from build123d import *

# Parameters (mm, degrees)
SKETCH2_R           = 5.9
BOSS_EXTRUDE1_DEPTH = 10
SKETCH3_R           = 2.075
CUT_EXTRUDE1_DEPTH  = 11
SKETCH4_W           = 11.8
SKETCH4_H           = 1
CUT_EXTRUDE2_DEPTH  = 11
CIRPATTERN1_COUNT   = 2
CIRPATTERN1_ANGLE   = 120


with BuildPart() as part:
    # Sketch2 → Boss-Extrude1 (new body)
    with BuildSketch(Plane(origin=(0, 0, 0), x_dir=(1, 0, 0), z_dir=(0, 1, 0))):
        Circle(SKETCH2_R)
    extrude(amount=BOSS_EXTRUDE1_DEPTH)

    # Sketch3 → Cut-Extrude1 (cut, through all)
    with BuildSketch(Plane(origin=(0, 10, 0), x_dir=(1, 0, 0), z_dir=(0, 1, 0))):
        Circle(SKETCH3_R)
    extrude(amount=-CUT_EXTRUDE1_DEPTH, mode=Mode.SUBTRACT)

    # Sketch4 → Cut-Extrude2 (cut, through all)
    with BuildSketch(Plane(origin=(0, 10, 0), x_dir=(1, 0, 0), z_dir=(0, 1, 0))):
        with Locations((0, 5.9)):
            Rectangle(SKETCH4_W, SKETCH4_H)
    cut_extrude2 = extrude(amount=-CUT_EXTRUDE2_DEPTH, mode=Mode.SUBTRACT)

    # CirPattern1: Cut-Extrude2 ×2 about axis
    cirpattern1_axis = Axis((0, 10, 0), (0, 1, 0))
    for i in range(1, CIRPATTERN1_COUNT):
        add(cut_extrude2.rotate(cirpattern1_axis, i * CIRPATTERN1_ANGLE / (CIRPATTERN1_COUNT - 1)), mode=Mode.SUBTRACT)


solid = part.part
The model under review builds one solid part; all positions refer to its coordinate system, in mm. Coordinates: 2 decimals unless noted, no trailing zeros. Loops run counter-clockwise (first coordinate to the right, second up) from the corner with the lowest first, then second, coordinate; pieces in that order, holes last. Notation, with made-up numbers: (70, -37) -> (108, -37) arc R24 ccw to (108, -24) -> close; hole circle Ø9 at (30, 51). An arc over 180 degrees is marked (long way). Use a Markdown table: item, result. Add a question column.
1. Add section A-A on x = 0. Write out the cut boundary in (y, z) (3 decimals).
2. Add section C-C on y = 6.5. Write out the cut boundary in (x, z) (3 decimals), plus the area to 3 significant figures.
3. Draft analysis for pull direction X (two halves, no side actions). For faces 1 (the face through (5.04, 4.93, 3.07)), 2 (the face through (-5.08, 4.93, -3)), 3 (the face through (0, 5, -5.4)), 4 (the face through (-0.45, 5.07, 2.026)), state which applies: pulls with the +X half, pulls with the -X half, needs draft (parallel to the pull), parting line crosses it, or undercut.
4. Add section B-B on z = 0. Write out the cut boundary in (x, y) (3 decimals), plus the area to 3 significant figures.
5. To check wall thickness, follow line 1 (Z direction, x = 0, y = 5.25) (3 decimals); line 2 (X direction, y = 3.5, z = 0) (3 decimals); line 3 (Z direction, x = 1.5, y = 7.5). State the ranges of each line that lie inside material, in increasing order.
6. Add section D-D on x = -4.5. Write out the cut boundary in (y, z), plus the area to 3 significant figures.
7. Clearance check with flat-ended pins moving along their axes: pin 1 Ø6 at (x, y) = (4, 7.5) entering from +Z; pin 2 Ø3.5 at (x, z) = (0, 0) entering from -Y. State where each tip first meets the part, or that it passes through.
Returned:
| question | item | result |
|---|---|---|
| 1 | outline | (0, -5.4) -> (10, -5.4) -> (10, -2.075) -> (0, -2.075) -> close; (0, 2.075) -> (10, 2.075) -> (10, 5.9) -> (0, 5.9) -> close |
| 2 | outline | (-5.865, 0.641) arc R5.9 ccw to (-2.377, -5.4) -> (2.377, -5.4) arc R5.9 ccw (long way) to (-3.488, 4.759) -> close; hole circle Ø4.15 at (0, 0) |
| 2 | area | 92.6 mm² |
| 3 | face 1 | parting line crosses it |
| 3 | face 2 | pulls with the -X half |
| 3 | face 3 | needs draft |
| 3 | face 4 | undercut |
| 4 | outline | (-5.9, 0) -> (-2.075, 0) -> (-2.075, 10) -> (-5.9, 10) -> close; (2.075, 0) -> (5.9, 0) -> (5.9, 10) -> (2.075, 10) -> close |
| 4 | area | 76.5 mm² |
| 5 | line 1 | z = -5.4 to -2.075, 2.075 to 5.9 |
| 5 | line 2 | x = -5.9 to -2.075, 2.075 to 5.9 |
| 5 | line 3 | z = -5.4 to -1.43, 1.43 to 5.71 |
| 6 | outline | (0, -3.82) -> (10, -3.82) -> (10, 3.01) -> (0, 3.01) -> close |
| 6 | area | 68.2 mm² |
| 7 | pin 1 | stops at z = 5.81 |
| 7 | pin 2 | passes through |
